Autodesk Inventor part; units mm, degrees
ref_plane "YZ Plane" through (0, 0, 0) normal (1, 0, 0) x (0, 1, 0)
ref_plane "XZ Plane" through (0, 0, 0) normal (0, 1, 0) x (-1, 0, 0)
ref_plane "XY Plane" through (0, 0, 0) normal (0, 0, 1) x (1, 0, 0)
sketch "Náčrt1" plane through (0, 0, 0) normal (0, 1, 0) x (-1, 0, 0)
  circle A0 centre (0, 0) radius 8
  line L0 (0, -8) -> (-50, -8)
  line L1 (-50, -8) -> (-50, 8)
  line L2 (-50, 8) -> (0, 8)
  circle A1 centre (0, 0) radius 3
  circle A2 centre (0, 0) radius 7.5 construction
  dimension "d0" = 6
  dimension "d1" = 15
  dimension "d2" = 16
  dimension "d3" = 50
extrude "Vysunutí1" add sketch "Náčrt1" along normal blind 6
sketch "Náčrt2" plane through (0, 6, 0) normal (0, 1, 0) x (1, 0, 0)
  line L0 (0, -8) -> (50, -8)
  line L1 (50, -8) -> (50, 8)
  line L2 (50, 8) -> (0, 8)
  arc A0 (0, 8) -> (0, -8) centre (0, 0) ccw
  circle A1 centre (0, 0) radius 3
  circle A2 centre (45, 0) radius 1.6
  circle A3 centre (25, 0) radius 1.6
  dimension "d6" = 5
  dimension "d7" = 25
  dimension "d8" = 3.2
extrude "Vysunutí2" cut sketch "Náčrt2" against normal through all contours A2 | A3
sketch "Náčrt5" plane through (0, 6, 0) normal (0, 1, 0) x (1, 0, 0)
  circle A0 centre (45, 0) radius 1.6
  circle A1 centre (25, 0) radius 1.6
  line L0 (0, -8) -> (50, -8)
  line L1 (50, -8) -> (50, 8)
  line L2 (50, 8) -> (0, 8)
  arc A2 (0, 8) -> (0, -8) centre (0, 0) ccw
  circle A3 centre (0, 0) radius 3
  line L3 (20, 8) -> (20, -8)
  dimension "d19" = 30
extrude "Vysunutí5" add sketch "Náčrt5" along normal blind 7 contours L3 L2 L1 L0
sketch "Náčrt7" plane through (0, 13, 0) normal (0, 1, 0) x (1, 0, 0)
  line L0 (50, 8) -> (20, 8)
  line L1 (20, 8) -> (20, -8)
  line L2 (20, -8) -> (50, -8)
  line L3 (50, -8) -> (50, 8)
  circle A0 centre (25, 0) radius 1.6
  circle A1 centre (45, 0) radius 1.6
  circle A2 centre (25, 0) radius 1.6
  circle A3 centre (25, 0) radius 3
  circle A4 centre (45, 0) radius 1.6
  circle A5 centre (45, 0) radius 3
  point P0 (0, 0)
  dimension "d22" = 6
extrude "Vysunutí6" cut sketch "Náčrt7" against normal blind 3 contours A3 | A5
sketch "Sketch10" plane through (20, 6, -8) normal (-1, 0, 0) x (0, 0, 1)
  line L0 (16, 0) -> (0, 0)
  line L1 (16, 0) -> (16, 7)
  line L2 (0, 7) -> (16, 7)
  line L3 (0, 0) -> (0, 7)
  point P0 (8, -6)
extrude "Extrusion8" add sketch "Sketch10" along normal blind 10
chamfer "Chamfer3" distance 0.5 angle 45 21 edges at (5, 6, 8) (-8, 6, 0) (5, 6, -8) (25, 0, 8) (-8, 0, 0) (25, 0, -8) (10, 13, 0) (30, 13, 8) (10, 9.5, 8) (30, 13, -8) (50, 13, 0) (42, 13, 0) (22, 13, 0) (3, 6, 0) (50, 0, 0) (50, 6.5, -8) (50, 6.5, 8) (10, 9.5, -8) (3, 0, 0) (23.4, 0, 0) (43.4, 0, 0)
properties part number "middle_joint"
Geometry check sheet. Reference: the model listing, model coordinates, mm. A direction names the side the tool comes from. Give positions to 0.01 mm unless a question says otherwise; leave off trailing zeros. Write each loop counter-clockwise with the first axis right and the second up, starting at its lowest first coordinate (ties: lowest second). Pieces come first, ordered by that corner, then holes. Notation, with made-up numbers: (54.5, 9) -> (85.5, 9) arc R33 cw to (85.5, 43) -> close; hole circle Ø11 at (64.25, -18). An arc over 180 degrees is marked (long way). Use one line per item in the form item = value.
Item 1: Mould release check, pull along X, two halves, no side actions. Record for faces 1 (the conical face through (-7.64, 5.86, 0.17)), 2 (the cylindrical face through (42, 11, 0)), 3 (the flat face through (50, 6, 0)): released by +X, released by -X, zero draft, split by the parting line, or undercut.
Results list:
face_1 = released by -X
face_2 = undercut
face_3 = released by +X
Item 2: Depth check by flat-ended pin: pin 1 Ø3 at (x, z) = (26, 1) entering from +Y; pin 2 Ø1.5 at (x, z) = (3.5, 3) entering from +Y; pin 3 Ø5 at (y, z) = (10, -1.5) entering from -X; pin 4 Ø1 at (x, z) = (37, -4.5) entering from -Y. Enter the tip coordinate at first touch or a pass-through.
Results list:
pin_1 = 10
pin_2 = 6
pin_3 = 10
pin_4 = 0
Item 3: Sectioned sample at C-C on y = 2.5. Enter the section's corners in (x, z), plus the area to 3 significant figures.
Results list:
outline = (0, -8) -> (49.5, -8) -> (50, -7.5) -> (50, 7.5) -> (49.5, 8) -> (0, 8) arc R8 ccw to start; hole circle Ø6 at (0, 0); hole circle Ø3.2 at (25, 0); hole circle Ø3.2 at (45, 0)
area = 856 mm2
Item 4: Sectioned sample at B-B on y = 6.5. Enter the section's corners in (x, z), plus the area to 3 significant figures.
Results list:
outline = (10, -7.5) -> (10.5, -8) -> (49.5, -8) -> (50, -7.5) -> (50, 7.5) -> (49.5, 8) -> (10.5, 8) -> (10, 7.5) -> close; hole circle Ø3.2 at (25, 0); hole circle Ø3.2 at (45, 0)
area = 623 mm2
Item 5: Sectioned sample at A-A on x = 45. Enter the section's corners in (y, z), plus the area to 3 significant figures.
Results list:
outline = (0, -7.5) -> (0.5, -8) -> (12.5, -8) -> (13, -7.5) -> (13, -3.5) -> (12.5, -3) -> (10, -3) -> (10, -1.6) -> (0.5, -1.6) -> (0, -2.1) -> close; (0, 2.1) -> (0.5, 1.6) -> (10, 1.6) -> (10, 3) -> (12.5, 3) -> (13, 3.5) -> (13, 7.5) -> (12.5, 8) -> (0.5, 8) -> (0, 7.5) -> close
area = 157 mm2
Item 6: Scan lines: line 1 (X direction, y = 11.6, z = 0); line 2 (X direction, y = 8.25, z = 0); line 3 (Z direction, x = 45, y = 10.95). Record each from-to range of solid material in increasing order.
Results list:
line_1 = 10 to 22, 28 to 42, 48 to 50
line_2 = 10 to 23.4, 26.6 to 43.4, 46.6 to 50
line_3 = -8 to -3, 3 to 8
Item 7: Access from +Z, -Z, +X, -X, +Y, -Y to the whole of each face (thin tool, end or side, straight path). Record for faces 4 (the flat face through (3.3, 6, 1.8)), 5 (the flat face through (25, 6, -8)), 6 (the flat face through (26.3, 10, 1.3)).
Results list:
face_4 = +Z, -Z, -X, +Y
face_5 = -Z, +X, -X, +Y, -Y
face_6 = +Y
Item 8: Sectioned sample at D-D on z = 0. Count the separate pieces of the cut face and the enclosed holes in it, plus the area to 3 significant figures.
Results list:
separate_pieces = 4
enclosed_holes = 0
area = 490 mm2
